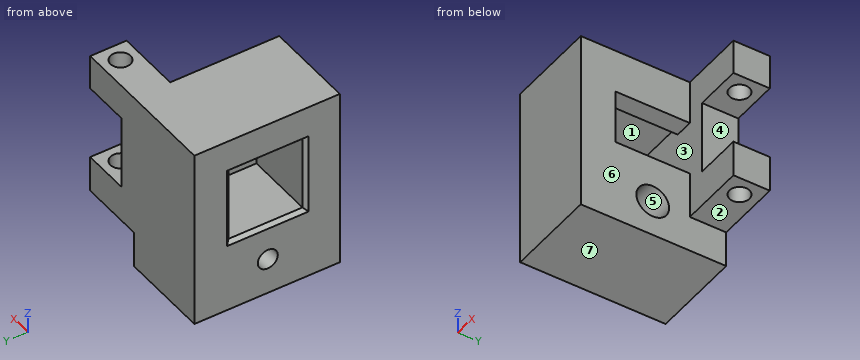
```python
from build123d import *

# Parameters (mm, degrees)
PAD_DEPTH        = 50
SKETCH001_W      = 13
SKETCH001_H      = 20.4
SKETCH001_W_2    = 18
SKETCH001_H_2    = 10
POCKET_DEPTH     = 10.001
SKETCH002_W      = 20.4
SKETCH002_H      = 20.4
POCKET001_DEPTH  = 20
SKETCH003_W      = 20.4
SKETCH003_H      = 15
POCKET002_DEPTH  = 5
HOLE_D           = 5.5
HOLE_CBORE_D     = 9
HOLE_CBORE_DEPTH = 20
SKETCH005_R      = 2.75
HOLE001_DEPTH    = 50.001
CHAMFER_SIZE     = 1


with BuildPart() as part:
    # Sketch → Pad (new body)
    with BuildSketch(Plane.XY):
        Polygon((0, 0), (18, 0), (18, 10), (-25, 10), (-25, -30), (0, -30), align=None)
    extrude(amount=PAD_DEPTH)

    # Sketch001 → Pocket (cut, through all)
    with BuildSketch(Plane.XZ):
        with Locations((11.5, 30.2)):
            Rectangle(SKETCH001_W, SKETCH001_H)
        with Locations((9, 5)):
            Rectangle(SKETCH001_W_2, SKETCH001_H_2)
    extrude(amount=-POCKET_DEPTH, mode=Mode.SUBTRACT)

    # Sketch002 (on Face12 of Pocket) → Pocket001 (cut)
    with BuildSketch(Plane(origin=(-25, 0, 0), x_dir=(0, -1, 0), z_dir=(-1, 0, 0))):
        with Locations((10.2, 30.2)):
            Rectangle(SKETCH002_W, SKETCH002_H)
    extrude(amount=-POCKET001_DEPTH, mode=Mode.SUBTRACT)

    # Sketch003 → Pocket002 (cut)
    with BuildSketch(Plane.YZ):
        with Locations((-10.2, 30.4)):
            Rectangle(SKETCH003_W, SKETCH003_H)
    extrude(amount=-POCKET002_DEPTH, mode=Mode.SUBTRACT)

    # Hole (through all)
    with Locations(Plane.YZ):
        with Locations((-10.2, 10)):
            CounterBoreHole(HOLE_D / 2, HOLE_CBORE_D / 2, HOLE_CBORE_DEPTH)

    # Sketch005 → Hole001 (cut, through all)
    with BuildSketch(Plane.XY):
        with Locations((13, 5)):
            Circle(SKETCH005_R)
    extrude(amount=HOLE001_DEPTH, mode=Mode.SUBTRACT)

    # Chamfer
    chamfer_edges = [part.edges().sort_by_distance(p)[0] for p in [
        (-25, -10.2, 40.4),
        (-25, 0, 30.2),
        (-25, -10.2, 20),
        (-25, -20.4, 30.2),
    ]]
    chamfer(chamfer_edges, length=CHAMFER_SIZE)


solid = part.part
```
Verification items for the finished model (mm, model axes). Face numbers are marked on the shaded views. A direction names the side the tool comes from. Coordinates: 2 decimals unless noted, no trailing zeros. Loops run counter-clockwise (first coordinate to the right, second up) from the corner with the lowest first, then second, coordinate; pieces in that order, holes last. Notation, with made-up numbers: (85.25, -23.75) -> (125.25, -23.75) arc R16 cw to (125.25, -5.75) -> close; hole circle Ø4 at (-2.5, 51). An arc over 180 degrees is marked (long way). Put each result on its own line as item: value.
1. Tool access check on the marked faces 1, 2, 3 and 4. Record the directions out of +Z, -Z, +X, -X, +Y, -Y that give a thin tool (end or side, any length) a straight path to the whole face; none if there is none.
Result set:
face 1: -X
face 2: -Z, +X, +Y, -Y
face 3: none
face 4: +X, +Y, -Y
2. Section check A-A, the plane x = -13. Record the boundary of the cut face in (y, z).
Result set:
outline: (-30, 0) -> (10, 0) -> (10, 50) -> (-30, 50) -> close; hole (-20.4, 20) -> (0, 20) -> (0, 40.4) -> (-20.4, 40.4) -> close; hole circle Ø9 at (-10.2, 10)
3. Gauge pin test, flat ends, axial feed: P1, Ø5.5, axis at x = -10, y = -5.5, coming from the -Z side; P2, Ø3, axis at x = 7, y = 6.5, coming from the -Z side; P3, Ø5, axis at y = 5.5, z = 33.5, coming from the +X side; P4, Ø7, axis at y = -12, z = 10.5, coming from the +X side. Record the tip position at first contact, or that the pin passes through.
Result set:
P1: stops at z = 0
P2: stops at z = 10
P3: stops at x = 5
P4: stops at x = 0
4. Section check D-D, the plane x = 13. Record the boundary of the cut face in (y, z).
Result set:
outline: (0, 10) -> (2.25, 10) -> (2.25, 20) -> (0, 20) -> close; (0, 40.4) -> (2.25, 40.4) -> (2.25, 50) -> (0, 50) -> close; (7.75, 10) -> (10, 10) -> (10, 20) -> (7.75, 20) -> close; (7.75, 40.4) -> (10, 40.4) -> (10, 50) -> (7.75, 50) -> close
5. Thickness scan on line 1 (Z direction, x = -21.65, y = -10.2); line 2 (X direction, y = 5, z = 17); line 3 (Z direction, x = -6.25, y = -10.2). Record the ranges inside material, lowest first.
Result set:
line 1: z = 0 to 7.25, 12.75 to 20, 40.4 to 50
line 2: x = -25 to 10.25, 15.75 to 18
line 3: z = 0 to 5.5, 14.5 to 20, 40.4 to 50
6. Section check B-B, the plane y = -10.2. Record the boundary of the cut face in (x, z).
Result set:
outline: (-25, 0) -> (0, 0) -> (0, 5.5) -> (-20, 5.5) -> (-20, 7.25) -> (-25, 7.25) -> close; (-25, 12.75) -> (-20, 12.75) -> (-20, 14.5) -> (0, 14.5) -> (0, 22.9) -> (-5, 22.9) -> (-5, 20) -> (-24, 20) -> (-25, 19) -> close; (-25, 41.4) -> (-24, 40.4) -> (-5, 40.4) -> (-5, 37.9) -> (0, 37.9) -> (0, 50) -> (-25, 50) -> close
7. Section check C-C, the plane z = 39. Record the boundary of the cut face in (x, y), then the cut area to 3 significant figures.
Result set:
outline: (-25, -30) -> (0, -30) -> (0, 0) -> (5, 0) -> (5, 10) -> (-25, 10) -> (-25, 1) -> (-24, 0) -> (-5, 0) -> (-5, -20.4) -> (-24, -20.4) -> (-25, -21.4) -> close
area: 641 mm^2
8. Mould release check, pull along Z, two halves, no side actions. Record for the marked faces 5, 6 and 7: pulls with the +Z half, pulls with the -Z half, needs draft (parallel to the pull), parting line crosses it, or undercut.
Result set:
face 5: undercut
face 6: needs draft
face 7: pulls with the -Z half
